Geometry check sheet. Reference: the model listing, model coordinates, mm. Round coordinates to 2 decimals unless told otherwise and drop trailing zeros. Write each loop counter-clockwise with the first axis right and the second up, starting at its lowest first coordinate (ties: lowest second). Pieces come first, ordered by that corner, then holes. Notation, with made-up numbers: M -36,-26.75 L 19,-26.75 A8 ccw 19,-12.75 Z; hole C 79.5,33 d6. An arc over 180 degrees is marked long. Use a Markdown table: item, result.
Autodesk Inventor part; units mm, degrees
ref_plane "YZ Plane" through (0, 0, 0) normal (1, 0, 0) x (0, 1, 0)
ref_plane "XZ Plane" through (0, 0, 0) normal (0, 1, 0) x (-1, 0, 0)
ref_plane "XY Plane" through (0, 0, 0) normal (0, 0, 1) x (1, 0, 0)
sketch "Sketch1" plane through (0, 0, 0) normal (0, 0, 1) x (1, 0, 0)
  line L0 (-10.9665, 63.5108) -> (69.0335, 63.5108)
  line L1 (69.0335, 63.5108) -> (69.0335, -16.4892)
  line L2 (69.0335, -16.4892) -> (-10.9665, -16.4892)
  line L3 (-10.9665, -16.4892) -> (-10.9665, 63.5108)
  circle A0 centre (-0.9665, 53.5108) radius 4
  line L4 (29.0335, 63.5108) -> (29.0335, 23.5108)
  line L5 (-10.9665, 23.5108) -> (29.0335, 23.5108)
  circle A1 centre (59.0335, 53.5108) radius 4
  circle A2 centre (-0.9665, -6.4892) radius 4
  circle A3 centre (59.0335, -6.4892) radius 4
  circle A4 centre (29.0335, 23.5108) radius 13.25
  point P0 (0, 0)
  dimension "d0" = 80
  dimension "d1" = 80
  dimension "d2" = 8
  dimension "d3" = 10
  dimension "d4" = 10
  dimension "d7" = 26.5
extrude "Plate1" add sketch "Sketch1" along normal mid plane 2
extrude "Cut1" cut sketch "Sketch1" against normal mid plane 2 contours A4 L5 L4 | L4 L5 A4
equation "\"d8\" = Thickness"
equation "\"d5\" = Thickness"
equation "\"BendRadius\" = Thickness"
equation "\"BendReliefWidth\" = Thickness"
equation "\"BendReliefDepth\" = 0.5 * Thickness"
equation "\"CornerReliefSize\" = 4 * Thickness"
equation "\"MinimumRemnant\" = 2 * Thickness"
equation "\"TransitionRadius\" = BendRadius"
equation "\"JacobiRadiusSize\" = BendRadius"
equation "\"GapSize\" = Thickness"
properties part number "plate"
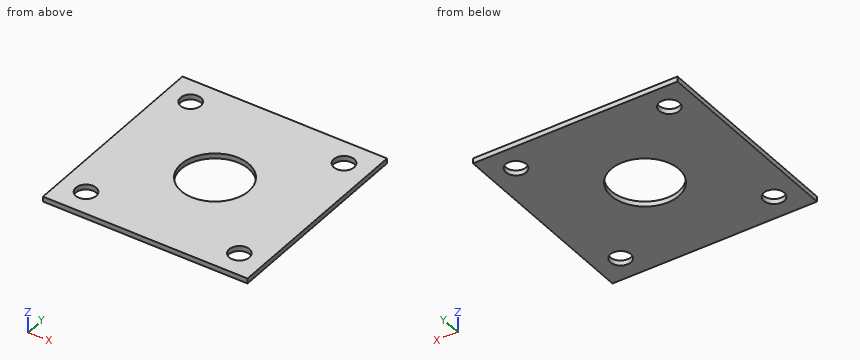
Item 1: Cross-section at A-A, the plane y = 35. Record the cut outline in (x, z).
Outcome:
| item | result |
|---|---|
| outline | M -10.97,-1 L 22.43,-1 L 22.43,1 L -10.97,1 Z; M 35.63,-1 L 69.03,-1 L 69.03,1 L 35.63,1 Z |
Item 2: Cross-section at B-B, the plane x = 2. Record the cut outline in (y, z), and give its area (3 significant figures).
Outcome:
| item | result |
|---|---|
| outline | M -16.49,-1 L -9.17,-1 L -9.17,1 L -16.49,1 Z; M -3.81,-1 L 50.83,-1 L 50.83,1 L -3.81,1 Z; M 56.19,-1 L 63.51,-1 L 63.51,1 L 56.19,1 Z |
| area | 139 mm2 |
Item 3: Cross-section at C-C, the plane x = 34.5. Record the cut outline in (y, z), and give its area (3 significant figures).
Outcome:
| item | result |
|---|---|
| outline | M -16.49,-1 L 11.44,-1 L 11.44,1 L -16.49,1 Z; M 35.58,-1 L 63.51,-1 L 63.51,1 L 35.58,1 Z |
| area | 112 mm2 |
Item 4: Material ranges on line 1 along Y through (x, z) = (-0.5, 0.8); line 2 along X through (y, z) = (56, 0.35); line 3 along X through (y, z) = (50, -0.35), recorded low to high. Write a range as from..to.
Outcome:
| item | result |
|---|---|
| line 1 | y = -16.49..-10.46, -2.52..49.54, 57.48..63.51 |
| line 2 | x = -10.97..-4.1, 2.16..55.9, 62.16..69.03 |
| line 3 | x = -10.97..-2.88, 0.95..57.12, 60.95..69.03 |
Item 5: Cross-section at D-D, the plane z = 0.4. Record the cut outline in (x, y), and give its area (3 significant figures).
Outcome:
| item | result |
|---|---|
| outline | M -10.97,-16.49 L 69.03,-16.49 L 69.03,63.51 L -10.97,63.51 Z; hole C -0.97,-6.49 d8; hole C -0.97,53.51 d8; hole C 29.03,23.51 d26.5; hole C 59.03,-6.49 d8; hole C 59.03,53.51 d8 |
| area | 5,650 mm2 |
